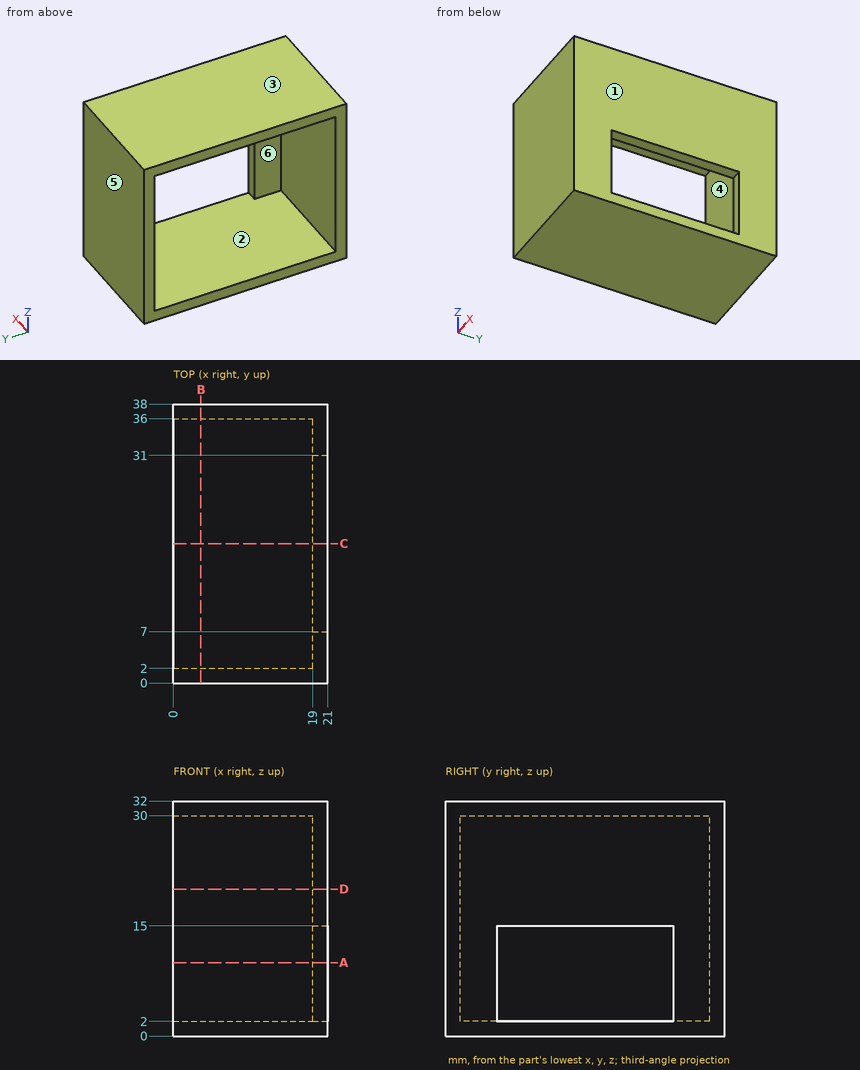
Study the drawing (mm; zero at the part's minimum x, y, z) and answer. A direction names the side the tool comes from. Give positions to 0.01 mm unless a question says otherwise; leave off trailing zeros. Loops run counter-clockwise (first coordinate to the right, second up) from the corner with the lowest first, then second, coordinate; pieces in that order, holes last. Notation, with made-up numbers: M -31,-0.75 L -9,-0.75 A17 ccw -9,11.25 Z; hole C 38.25,64 d4. An arc over 180 degrees is marked long. Answer as CSV lines item,"result".
Item 1: The part is cut by section A-A (z = 10). Give the vertices of the cut face in (x, y), and give its area (3 significant figures).
Values follow:
outline,"M 0,0 L 21,0 L 21,7 L 19,7 L 19,2 L 0,2 Z; M 0,36 L 19,36 L 19,31 L 21,31 L 21,38 L 0,38 Z"
area,"104 mm^2"
Item 2: The mould has two halves that part along Y. Classify the marked faces 3, 4, 5 and 6: released by +Y, released by -Y, zero draft, split by the parting line, or undercut.
Values follow:
face 3,"zero draft"
face 4,"undercut"
face 5,"released by +Y"
face 6,"undercut"
Item 3: The part is cut by section D-D (z = 20). Give the vertices of the cut face in (x, y), and give its area (3 significant figures).
Values follow:
outline,"M 0,0 L 21,0 L 21,38 L 0,38 L 0,36 L 19,36 L 19,2 L 0,2 Z"
area,"152 mm^2"
Item 4: The part is cut by section B-B (x = 3.75). Give the vertices of the cut face in (y, z).
Values follow:
outline,"M 0,0 L 38,0 L 38,32 L 0,32 Z; hole M 2,2 L 36,2 L 36,30 L 2,30 Z"
Item 5: Straight lines are drawn through the part: line 1 along Z through (x, y) = (1.25, 22); line 2 along Y through (x, z) = (6, 2.5); line 3 along Y through (x, z) = (20.25, 3.5). For each, find the intervals that lie inside material, in ascending order. Write a range as [from, to].
Values follow:
line 1,"z = [0, 2], [30, 32]"
line 2,"y = [0, 2], [36, 38]"
line 3,"y = [0, 7], [31, 38]"
Item 6: Given pin 1 Ø4 at (x, z) = (3, 15) entering from -Y; pin 2 Ø6 at (y, z) = (27, 11.5) entering from -X; pin 3 Ø10 at (y, z) = (7.5, 16.5) entering from -X, each flat-ended and moving along its own axis, determine where each tip first touches the part or whether it passes through.
Values follow:
pin 1,"stops at y = 0"
pin 2,"passes through"
pin 3,"stops at x = 19"
Item 7: Which of the six approach directions +Z, -Z, +X, -X, +Y, -Y give full straight-line access (tool end or side, diameter ignored) to the marked faces 1 and 2?
Values follow:
face 1,"+Z, -Z, +X, +Y, -Y"
face 2,"-X"
Item 8: The part is cut by section C-C (y = 19). Give the vertices of the cut face in (x, z), and give its area (3 significant figures).
Values follow:
outline,"M 0,0 L 21,0 L 21,2 L 0,2 Z; M 0,30 L 19,30 L 19,15 L 21,15 L 21,32 L 0,32 Z"
area,"114 mm^2"
